The model under review builds one solid part; all positions refer to its coordinate system, in mm. A direction names the side the tool comes from. Give positions to 0.01 mm unless a question says otherwise; leave off trailing zeros. Order: outer loops, then holes, each group sorted by start corner. A loop starts at its lowest first (then second) coordinate and runs counter-clockwise, first axis right, second up. Notation, with made-up numbers: (-36.5, 64.25) -> (-3.5, 64.25) arc R21 ccw to (-3.5, 70.25) -> close; hole circle Ø6 at (4.25, -28). An arc over 180 degrees is marked (long way). Answer as a JSON object with one key per item and string values. Group by question number.
from build123d import *

# Parameters (mm, degrees)
SKETCH026_W      = 8.25
SKETCH026_H      = 20
EXTRUDE031_DEPTH = 10
SKETCH023_R      = 4.125
EXTRUDE028_DEPTH = 60
SKETCH022_W      = 4
SKETCH022_H      = 64
EXTRUDE027_DEPTH = 26
SKETCH025_W      = 2
SKETCH025_H      = 20
EXTRUDE030_DEPTH = 20
SKETCH024_W      = 40
SKETCH024_H      = 64
EXTRUDE029_DEPTH = 2


with BuildPart() as extrude031:
    # Sketch026 (on Sketch) → Extrude031 (new body)
    with BuildSketch(Plane.YZ):
        with Locations((-19.875, 65.75)):
            Rectangle(SKETCH026_W, SKETCH026_H)
    extrude(amount=EXTRUDE031_DEPTH)


with BuildPart() as extrude031_1:
    # Extrude031 placement: moved
    add(extrude031.part.moved(Location((-21.5, 0.1, 0))))


with BuildPart() as fusion010:
    # Sketch023 → Extrude028 (new body)
    with BuildSketch(Plane.YZ):
        with Locations((-19.75, 55.75)):
            Circle(SKETCH023_R)
    extrude(amount=EXTRUDE028_DEPTH)


with BuildPart() as fusion010_1:
    # Extrude028 placement: moved
    add(fusion010.part.moved(Location((-21.5, 0, 0))))

    # Fusion010: union Extrude031
    add(extrude031_1.part)


with BuildPart() as extrude027:
    # Sketch022 → Extrude027 (new body, symmetric)
    with BuildSketch(Plane.XZ):
        with Locations((-22, 32)):
            Rectangle(SKETCH022_W, SKETCH022_H)
        with Locations((22, 32)):
            Rectangle(SKETCH022_W, SKETCH022_H)
    extrude(amount=EXTRUDE027_DEPTH, both=True)


with BuildPart() as extrude030:
    # Sketch025 → Extrude030 (new body, symmetric)
    with BuildSketch(Plane.YZ):
        with Locations((-23, 40)):
            Rectangle(SKETCH025_W, SKETCH025_H)
    extrude(amount=EXTRUDE030_DEPTH, both=True)


with BuildPart() as cut005:
    # Sketch024 → Extrude029 (new body)
    with BuildSketch(Plane.XZ):
        with Locations((0, 32)):
            Rectangle(SKETCH024_W, SKETCH024_H)
    extrude(amount=-EXTRUDE029_DEPTH)


with BuildPart() as cut005_1:
    # Extrude029 placement: moved
    add(cut005.part.moved(Location((0, 24, 0))))

    # Fusion011: union Extrude027, Extrude030
    add(extrude027.part)
    add(extrude030.part)

    # Cut005: cut Fusion010
    add(fusion010_1.part, mode=Mode.SUBTRACT)


solid = cut005_1.part
1. Draft analysis for pull direction Z (two halves, no side actions). For faces 1 (the flat face through (0, -23, 50)), 2 (the cylindrical face through (21.972, -20.644, 51.723)), 3 (the flat face through (-24, 0, 32)), state which applies: pulls with the +Z half, pulls with the -Z half, needs draft (parallel to the pull), parting line crosses it, or undercut.
2. Take a section at D-D on y = -19.75. Give the boundary of the cut face in (x, z) (3 decimals), plus the area to 3 significant figures.
3. Take a section at B-B on y = 6.5. Give the boundary of the cut face in (x, z).
4. Take a section at C-C on z = 25. Give the boundary of the cut face in (x, y).
5. Take a section at A-A on x = -4. Give the boundary of the cut face in (y, z), plus the area to 3 significant figures.
6. Machinability: for faces 4 (the flat face through (0, -22, 40)), 5 (the flat face through (0, -24, 40)), 6 (the flat face through (-21, -15.65, 60)), 7 (the flat face through (2, 25, 64)), which of the approach directions +Z, -Z, +X, -X, +Y, -Y give a long, thin tool a straight path to every point of the face, cutting with its end or side? Answer none if there is none.
7. For pin 1 (4 mm diameter, centred on x = 9, z = 15, fed in from -Y); pin 2 (10 mm diameter, centred on x = 10.5, y = 3.5, fed in from +Z); pin 3 (0.6 mm diameter, centred on x = -7.5, y = -22.5, fed in from -Z); pin 4 (16 mm diameter, centred on x = -1, z = 45, fed in from -Y), all flat-tipped, find the tip position at first contact; note any pin that passes through.
8. For probe 1 along X at (y, z) = (18, 45); probe 2 along Y at (x, z) = (12, 36); probe 3 along Z at (x, y) = (21.1, -19.75) (3 decimals), list the stretches that pass through material, from the lowest coordinate up. Write a range as [from, to].
Checks:
{
 "1": {"face 1": "pulls with the +Z half", "face 2": "undercut", "face 3": "needs draft"},
 "2": {"outline": "(-24, 0) -> (-20, 0) -> (-20, 51.625) -> (-21.5, 51.625) -> (-21.5, 64) -> (-24, 64) -> close; (20, 0) -> (24, 0) -> (24, 51.625) -> (20, 51.625) -> close; (20, 59.875) -> (24, 59.875) -> (24, 64) -> (20, 64) -> close", "area": "460 mm2"},
 "3": {"outline": "(-24, 0) -> (-20, 0) -> (-20, 64) -> (-24, 64) -> close; (20, 0) -> (24, 0) -> (24, 64) -> (20, 64) -> close"},
 "4": {"outline": "(-24, -26) -> (-20, -26) -> (-20, 24) -> (20, 24) -> (20, -26) -> (24, -26) -> (24, 26) -> (-24, 26) -> close"},
 "5": {"outline": "(-24, 30) -> (-22, 30) -> (-22, 50) -> (-24, 50) -> close; (24, 0) -> (26, 0) -> (26, 64) -> (24, 64) -> close", "area": "168 mm2"},
 "6": {"face 4": "+Z, -Z", "face 5": "+Z, -Z, -Y", "face 6": "+Z", "face 7": "+Z, +X, -X, +Y, -Y"},
 "7": {"pin 1": "stops at y = 24", "pin 2": "passes through", "pin 3": "stops at z = 30", "pin 4": "stops at y = -24"},
 "8": {"probe 1": "x = [-24, -20], [20, 24]", "probe 2": "y = [-24, -22], [24, 26]", "probe 3": "z = [0, 51.625], [59.875, 64]"}
}
